from build123d import *

# Parameters (mm, degrees)
SKETCH2_R           = 2.125
SKETCH2_R_2         = 11.5
BOSS_EXTRUDE2_DEPTH = 3


with BuildPart() as part:
    # Sketch2 → Boss-Extrude2 (new body)
    with BuildSketch(Plane.XY):
        with BuildLine():
            Line((-4.375, 23.324003444), (-4.375, 27.149758286))
            ThreePointArc((-4.375, 27.149758286), (-8.497967345, 26.154054198), (-12.418778174, 24.536176326))
            Line((-12.418778174, 24.536176326), (-10.170055898, 21.441075642))
            ThreePointArc((-10.170055898, 21.441075642), (-13.044413657, 17.954095121), (-17.248954599, 16.297954684))
            Line((-17.248954599, 16.297954684), (-19.497676874, 19.393055368))
            ThreePointArc((-19.497676874, 19.393055368), (-22.247967345, 16.164094438), (-24.469005184, 12.550608962))
            Line((-24.469005184, 12.550608962), (-20.830496111, 11.3683857))
            ThreePointArc((-20.830496111, 11.3683857), (-21.106304661, 6.857854099), (-23.534394812, 3.046641182))
            Line((-23.534394812, 3.046641182), (-27.172903884, 4.228864445))
            ThreePointArc((-27.172903884, 4.228864445), (-27.5, 0), (-27.172903884, -4.228864445))
            Line((-27.172903884, -4.228864445), (-23.534394812, -3.046641182))
            ThreePointArc((-23.534394812, -3.046641182), (-21.106304661, -6.857854099), (-20.830496111, -11.3683857))
            Line((-20.830496111, -11.3683857), (-24.469005184, -12.550608962))
            ThreePointArc((-24.469005184, -12.550608962), (-22.247967345, -16.164094438), (-19.497676874, -19.393055368))
            Line((-19.497676874, -19.393055368), (-17.248954599, -16.297954684))
            ThreePointArc((-17.248954599, -16.297954684), (-13.044413657, -17.954095121), (-10.170055898, -21.441075642))
            Line((-10.170055898, -21.441075642), (-12.418778174, -24.536176326))
            ThreePointArc((-12.418778174, -24.536176326), (-8.497967345, -26.154054198), (-4.375, -27.149758286))
            Line((-4.375, -27.149758286), (-4.375, -23.324003444))
            ThreePointArc((-4.375, -23.324003444), (0, -22.192482044), (4.375, -23.324003444))
            Line((4.375, -23.324003444), (4.375, -27.149758286))
            ThreePointArc((4.375, -27.149758286), (8.497967345, -26.154054198), (12.418778174, -24.536176326))
            Line((12.418778174, -24.536176326), (10.170055898, -21.441075642))
            ThreePointArc((10.170055898, -21.441075642), (13.044413657, -17.954095121), (17.248954599, -16.297954684))
            Line((17.248954599, -16.297954684), (19.497676874, -19.393055368))
            ThreePointArc((19.497676874, -19.393055368), (22.247967345, -16.164094438), (24.469005184, -12.550608962))
            Line((24.469005184, -12.550608962), (20.830496111, -11.3683857))
            ThreePointArc((20.830496111, -11.3683857), (21.106304661, -6.857854099), (23.534394812, -3.046641182))
            Line((23.534394812, -3.046641182), (27.172903884, -4.228864445))
            ThreePointArc((27.172903884, -4.228864445), (27.5, 0), (27.172903884, 4.228864445))
            Line((27.172903884, 4.228864445), (23.534394812, 3.046641182))
            ThreePointArc((23.534394812, 3.046641182), (21.106304661, 6.857854099), (20.830496111, 11.3683857))
            Line((20.830496111, 11.3683857), (24.469005184, 12.550608962))
            ThreePointArc((24.469005184, 12.550608962), (22.247967345, 16.164094438), (19.497676874, 19.393055368))
            Line((19.497676874, 19.393055368), (17.248954599, 16.297954684))
            ThreePointArc((17.248954599, 16.297954684), (13.044413657, 17.954095121), (10.170055898, 21.441075642))
            Line((10.170055898, 21.441075642), (12.418778174, 24.536176326))
            ThreePointArc((12.418778174, 24.536176326), (8.497967345, 26.154054198), (4.375, 27.149758286))
            Line((4.375, 27.149758286), (4.375, 23.324003444))
            ThreePointArc((4.375, 23.324003444), (0, 22.192482044), (-4.375, 23.324003444))
        make_face()
        with Locations((16.02146997, 9.25)):
            Circle(SKETCH2_R, mode=Mode.SUBTRACT)
        with Locations((0, 18.5)):
            Circle(SKETCH2_R, mode=Mode.SUBTRACT)
        with Locations((-16.02146997, 9.25)):
            Circle(SKETCH2_R, mode=Mode.SUBTRACT)
        with Locations((-16.02146997, -9.25)):
            Circle(SKETCH2_R, mode=Mode.SUBTRACT)
        with Locations((0, -18.5)):
            Circle(SKETCH2_R, mode=Mode.SUBTRACT)
        with Locations((16.02146997, -9.25)):
            Circle(SKETCH2_R, mode=Mode.SUBTRACT)
        Circle(SKETCH2_R_2, mode=Mode.SUBTRACT)
    extrude(amount=BOSS_EXTRUDE2_DEPTH)


solid = part.part
The model under review builds one solid part; all positions refer to its coordinate system, in mm. A direction names the side the tool comes from. Round coordinates to 2 decimals unless told otherwise and drop trailing zeros. Write each loop counter-clockwise with the first axis right and the second up, starting at its lowest first coordinate (ties: lowest second). Pieces come first, ordered by that corner, then holes. Notation, with made-up numbers: M 41,15.25 L 99,15.25 A11 cw 99,36.25 Z; hole C -1.75,76.5 d2. An arc over 180 degrees is marked long. Use a Markdown table: item, result. Add a question column.
Q1. The part is to be moulded in two halves that separate along X. For faces 1 (the face through (-13.096, -17.917, 1.479)), 2 (the face through (-8.441, 26.172, 1.479)), 3 (the face through (8.441, -26.172, 1.479)), say which applies: pulls with the +X half, pulls with the -X half, needs draft (parallel to the pull), parting line crosses it, or undercut.
Q2. We need section A-A, the plane y = 0. State the section outline as (x, z) points.
Q3. We need section B-B, the plane y = -18.5. State the section outline as (x, z) points (3 decimals), plus the area to 3 significant figures.
Q4. Machinability: for faces 4 (the face through (18.39, 17.87, 1.48)), 5 (the face through (12.993, -17.992, 1.479)), 6 (the face through (22.68, -11.97, 1.48)), which of the approach directions +Z, -Z, +X, -X, +Y, -Y give a long, thin tool a straight path to every point of the face, cutting with its end or side? Answer none if there is none.
Q5. Insertion check: pin 1 (0.9 mm diameter, centred on y = 25.5, z = 1, fed in from +X); pin 2 (1 mm diameter, centred on y = 4, z = 1.5, fed in from +X); pin 3 (4 mm diameter, centred on x = 0, y = 18.5, fed in from +Z). Each pin has a flat end and moves straight along its axis. Give the tip position at first contact, or say it passes through.
Q6. We need section D-D, the plane y = -8. State the section outline as (x, z) points, plus the area to 3 significant figures.
Q7. To check wall thickness, follow line 1 (Y direction, x = -16, z = 2.4); line 2 (Y direction, x = 1, z = 0.6) (3 decimals); line 3 (Y direction, x = -22.5, z = 1.1). State the ranges of each line that lie inside material, in increasing order.
Q8. We need section C-C, the plane z = 1.2. Count the separate pieces of the cut face and the enclosed holes in it, plus the area to 3 significant figures.
Findings below:
| question | item | result |
|---|---|---|
| 1 | face 1 | undercut |
| 1 | face 2 | pulls with the -X half |
| 1 | face 3 | pulls with the +X half |
| 2 | outline | M -27.5,0 L -11.5,0 L -11.5,3 L -27.5,3 Z; M 11.5,0 L 27.5,0 L 27.5,3 L 11.5,3 Z |
| 3 | outline | M -20.347,0 L -18.849,0 L -18.849,3 L -20.347,3 Z; M -12.365,0 L -2.125,0 L -2.125,3 L -12.365,3 Z; M 2.125,0 L 12.365,0 L 12.365,3 L 2.125,3 Z; M 18.849,0 L 20.347,0 L 20.347,3 L 18.849,3 Z |
| 3 | area | 70.4 mm² |
| 4 | face 4 | +Z, -Z, +Y |
| 4 | face 5 | +Z, -Z |
| 4 | face 6 | +Z, -Z, +X |
| 5 | pin 1 | stops at x = 11.35 |
| 5 | pin 2 | stops at x = 27.28 |
| 5 | pin 3 | passes through |
| 6 | outline | M -20.82,0 L -17.74,0 L -17.74,3 L -20.82,3 Z; M -14.3,0 L -8.26,0 L -8.26,3 L -14.3,3 Z; M 8.26,0 L 14.3,0 L 14.3,3 L 8.26,3 Z; M 17.74,0 L 20.82,0 L 20.82,3 L 17.74,3 Z |
| 6 | area | 54.7 mm² |
| 7 | line 1 | y = -16.54 to -11.37, -7.13 to 7.13, 11.37 to 16.54 |
| 7 | line 2 | y = -22.248 to -20.375, -16.625 to -11.456, 11.456 to 16.625, 20.375 to 22.248 |
| 7 | line 3 | y = -15.81 to -11.91, -4.19 to 4.19, 11.91 to 15.81 |
| 8 | separate pieces | 1 |
| 8 | enclosed holes | 7 |
| 8 | area | 1,450 mm² |
